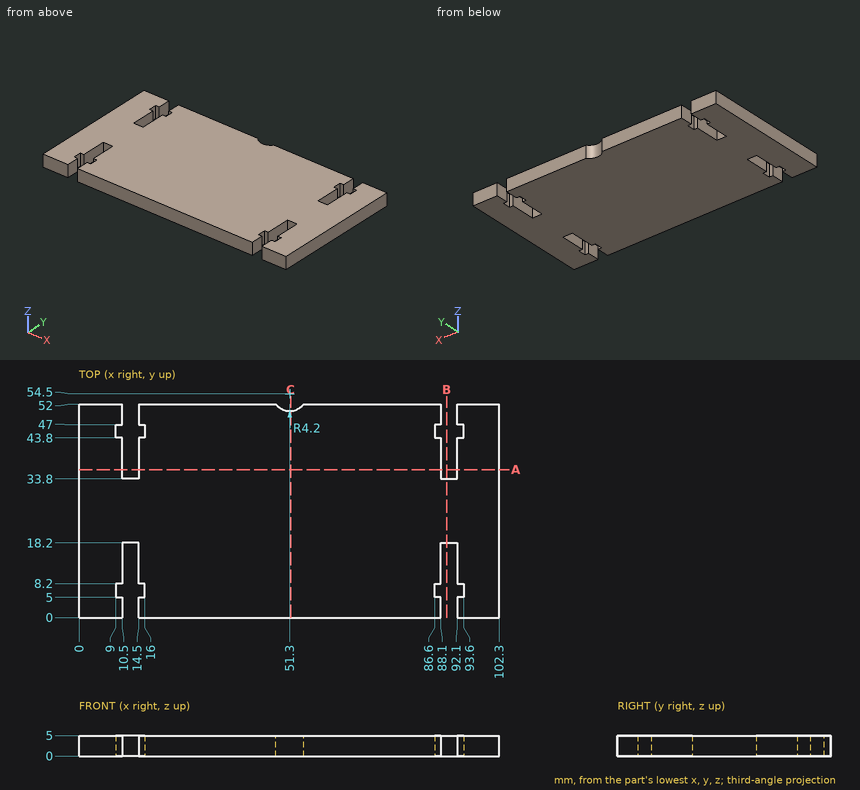
Verification items for this drawing (mm, ordinates from the low corner). Give positions to 0.01 mm unless a question says otherwise; leave off trailing zeros. Loops run counter-clockwise (first coordinate to the right, second up) from the corner with the lowest first, then second, coordinate; pieces in that order, holes last. Notation, with made-up numbers: M 14.25,44 L 58.25,44 A29 ccw 58.25,77 Z; hole C -6,6.5 d7. An arc over 180 degrees is marked long. Return JSON: item names as keys, results as strings. Group by question number.
1. Go/stop test with a flat-tipped pin: pin 1 (1 mm diameter, centred on x = 75.5, y = 26, fed in from -Z). Record where the tip stops, or that it passes through.
2. Cross-section at B-B on x = 89.5. Record the boundary of the cut face in (y, z), plus the area to 3 significant figures.
3. Thickness scan on L1, parallel to X at y = 44, z = 4.75; L2, parallel to X at y = 41.5, z = 1.8; L3, parallel to Y at x = 91, z = 0.75. Record the ranges inside material, lowest first.
4. Cross-section at A-A on y = 36. Record the boundary of the cut face in (x, z), plus the area to 4 significant figures.
5. Cross-section at C-C on x = 51.5. Record the boundary of the cut face in (y, z).
Return value:
{
 "1": {"pin 1": "z = 0"},
 "2": {"outline": "M 18.2,0 L 33.8,0 L 33.8,5 L 18.2,5 Z", "area": "78.0 mm^2"},
 "3": {"L1": "0 to 9, 16 to 86.6, 93.6 to 102.3", "L2": "0 to 10.5, 14.5 to 88.1, 92.1 to 102.3", "L3": "18.2 to 33.8"},
 "4": {"outline": "M 0,0 L 10.5,0 L 10.5,5 L 0,5 Z; M 14.5,0 L 88.1,0 L 88.1,5 L 14.5,5 Z; M 92.1,0 L 102.3,0 L 102.3,5 L 92.1,5 Z", "area": "471.5 mm^2"},
 "5": {"outline": "M 0,0 L 50.3,0 L 50.3,5 L 0,5 Z"}
}
